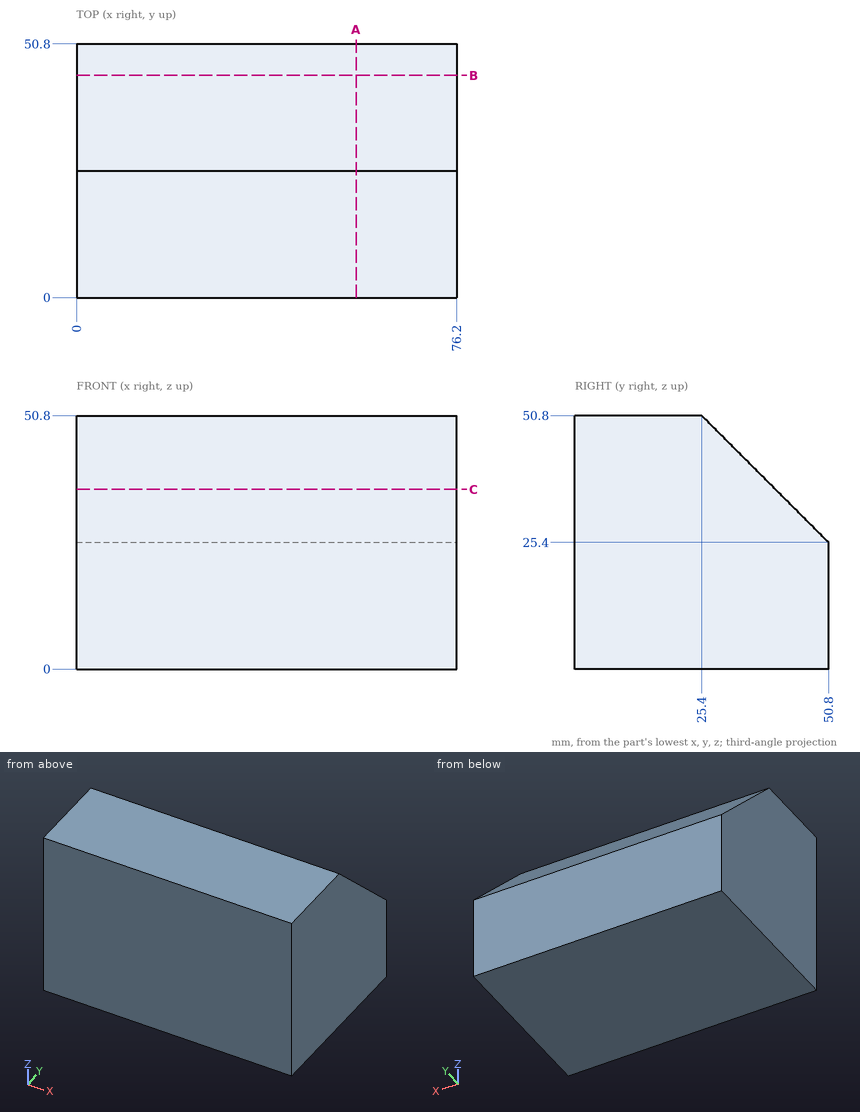
Design review of the part shown in the three views and the two pictorial views. Dimensions are in mm from the part's minimum x, y and z. Round coordinates to 2 decimals unless told otherwise and drop trailing zeros. Order: outer loops, then holes, each group sorted by start corner. A loop starts at its lowest first (then second) coordinate and runs counter-clockwise, first axis right, second up.
Q1. We need section B-B, the plane y = 44.5. Give the boundary of the cut face in (x, z).
Findings below:
outline: (0, 0) - (76.2, 0) - (76.2, 31.7) - (0, 31.7) - close
Q2. We need section A-A, the plane x = 56. Give the boundary of the cut face in (y, z), plus the area to 3 significant figures.
Findings below:
outline: (0, 0) - (50.8, 0) - (50.8, 25.4) - (25.4, 50.8) - (0, 50.8) - close
area: 2,260 mm2
Q3. We need section C-C, the plane z = 36. Give the boundary of the cut face in (x, y), plus the area to 3 significant figures.
Findings below:
outline: (0, 0) - (76.2, 0) - (76.2, 40.2) - (0, 40.2) - close
area: 3,060 mm2
Q4. Wall thickness on line 1 (Z direction, x = 39, y = 35.5); line 2 (Y direction, x = 13.5, z = 30); line 3 (Z direction, x = 25, y = 33.5): over which ranges is each line inside the solid? List them lowest first.
Findings below:
line 1: z = 0 to 40.7
line 2: y = 0 to 46.2
line 3: z = 0 to 42.7
